Check sheet for the modelled part. Datum: model origin and axes. Units: mm. Face numbers are marked on the shaded views. A direction names the side the tool comes from. Round coordinates to 2 decimals unless told otherwise and drop trailing zeros. Write each loop counter-clockwise with the first axis right and the second up, starting at its lowest first coordinate (ties: lowest second). Pieces come first, ordered by that corner, then holes.
Item 1: Release check for a two-part mould opening along X. For the marked faces 3 and 4 record: pulls with the +X half, pulls with the -X half, needs draft (parallel to the pull), parting line crosses it, or undercut.
Item 2: Section check A-A, the plane z = 4. Record the cut outline in (x, y).
Item 3: Material ranges on line 1 along X through (y, z) = (7, 5.25); line 2 along X through (y, z) = (7, 5.5); line 3 along Y through (x, z) = (-4.5, 3), recorded low to high.
Item 4: Set-up check for the marked faces 1 and 2: record each of +Z, -Z, +X, -X, +Y, -Y from which the full face is reachable in a straight line by a thin tool's end or side.
Item 5: Section check B-B, the plane y = 13. Record the cut outline in (x, z).
Item 6: Depth check by flat-ended pin: pin 1 (1.5 mm diameter, centred on x = 15.5, z = 5, fed in from +Y); pin 2 (1.5 mm diameter, centred on x = -9.5, y = -23.5, fed in from -Z); pin 3 (1.5 mm diameter, centred on y = 1, z = 2, fed in from -X). Enter the tip coordinate at first touch or a pass-through.
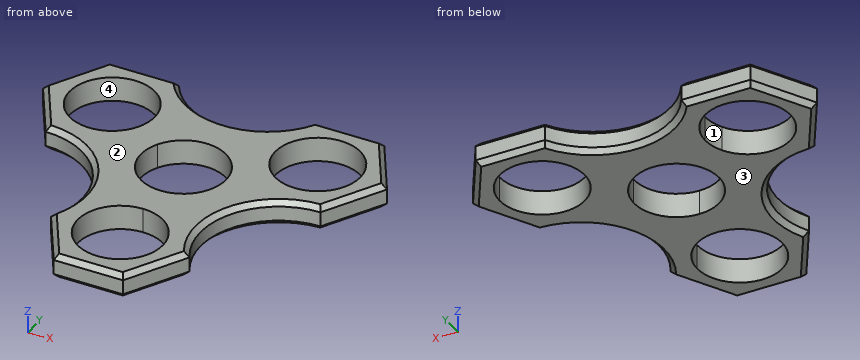
from build123d import *

# Parameters (mm, degrees)
F1_DEPTH = 6.35
F2_SIZE  = 1.27
F3_SIZE  = 1.27


with BuildPart() as f1:
    # F0 (on Top) → F1 (new body)
    with BuildSketch(Plane.XY):
        with BuildLine():
            ThreePointArc((9.535719, 5.50545), (10.635713, 2.849831), (11.0109, 0))
            ThreePointArc((11.0109, 0), (7.785882, -7.785882), (0, -11.0109))
            Line((0, -11.0109), (0, -15.082068))
            Line((0, -15.082068), (8.89, -15.082068))
            Line((8.89, -15.082068), (17.78, -30.48))
            ThreePointArc((17.78, -30.48), (17.78, -10.265288), (35.286454, -0.157932))
            Line((35.286454, -0.157932), (17.506454, -0.157932))
            Line((17.506454, -0.157932), (13.061454, 7.541034))
            Line((13.061454, 7.541034), (9.535719, 5.50545))
        make_face()
        with BuildLine():
            ThreePointArc((-9.535719, 5.50545), (0, 11.0109), (9.535719, 5.50545))
            Line((9.535719, 5.50545), (13.061454, 7.541034))
            Line((13.061454, 7.541034), (8.616454, 15.24))
            Line((8.616454, 15.24), (17.506454, 30.637932))
            ThreePointArc((17.506454, 30.637932), (0, 20.530576), (-17.506454, 30.637932))
            Line((-17.506454, 30.637932), (-8.616454, 15.24))
            Line((-8.616454, 15.24), (-13.061454, 7.541034))
            Line((-13.061454, 7.541034), (-9.535719, 5.50545))
        make_face()
        with BuildLine():
            Line((0, -15.082068), (0, -11.0109))
            ThreePointArc((0, -11.0109), (-9.535719, -5.50545), (-9.535719, 5.50545))
            Line((-9.535719, 5.50545), (-13.061454, 7.541034))
            Line((-13.061454, 7.541034), (-17.506454, -0.157932))
            Line((-17.506454, -0.157932), (-35.286454, -0.157932))
            ThreePointArc((-35.286454, -0.157932), (-17.78, -10.265288), (-17.78, -30.48))
            Line((-17.78, -30.48), (-8.89, -15.082068))
            Line((-8.89, -15.082068), (0, -15.082068))
        make_face()
        with BuildLine():
            ThreePointArc((37.407354, 15.24), (23.546624, 25.875713), (16.860735, 9.73455))
            ThreePointArc((16.860735, 9.73455), (29.246285, 4.604287), (37.407354, 15.24))
        make_face()
        Polygon((8.616454, 15.24), (13.061454, 7.541034), (17.506454, -0.157932), (35.286454, -0.157932), (44.176454, 15.24), (35.286454, 30.637932), (17.506454, 30.637932), align=None)
        with BuildLine():
            ThreePointArc((37.407354, 15.24), (29.246285, 4.604287), (16.860735, 9.73455))
            ThreePointArc((16.860735, 9.73455), (23.546624, 25.875713), (37.407354, 15.24))
        make_face(mode=Mode.SUBTRACT)
        with BuildLine():
            ThreePointArc((11.0109, -30.48), (7.785882, -22.694118), (0, -19.4691))
            ThreePointArc((0, -19.4691), (-7.785882, -38.265882), (11.0109, -30.48))
        make_face()
        Polygon((8.89, -15.082068), (0, -15.082068), (-8.89, -15.082068), (-17.78, -30.48), (-8.89, -45.877932), (8.89, -45.877932), (17.78, -30.48), align=None)
        with BuildLine():
            ThreePointArc((11.0109, -30.48), (-7.785882, -38.265882), (0, -19.4691))
            ThreePointArc((0, -19.4691), (7.785882, -22.694118), (11.0109, -30.48))
        make_face(mode=Mode.SUBTRACT)
        with BuildLine():
            ThreePointArc((-15.385554, 15.24), (-37.032167, 18.089831), (-16.860735, 9.73455))
            ThreePointArc((-16.860735, 9.73455), (-15.760742, 12.390169), (-15.385554, 15.24))
        make_face()
        Polygon((-17.506454, -0.157932), (-13.061454, 7.541034), (-8.616454, 15.24), (-17.506454, 30.637932), (-35.286454, 30.637932), (-44.176454, 15.24), (-35.286454, -0.157932), align=None)
        with BuildLine():
            ThreePointArc((-15.385554, 15.24), (-15.760742, 12.390169), (-16.860735, 9.73455))
            ThreePointArc((-16.860735, 9.73455), (-37.032167, 18.089831), (-15.385554, 15.24))
        make_face(mode=Mode.SUBTRACT)
    extrude(amount=F1_DEPTH)

    # F2
    f2_edges = [f1.edges().sort_by_distance(p)[0] for p in [
        (-26.396454, 30.637932, 6.35),
        (0, 20.530576, 6.35),
        (26.396454, 30.637932, 6.35),
        (39.731454, 22.938966, 6.35),
        (39.731454, 7.541034, 6.35),
        (17.78, -10.265288, 6.35),
        (13.335, -38.178966, 6.35),
        (0, -45.877932, 6.35),
        (-13.335, -38.178966, 6.35),
        (-17.78, -10.265288, 6.35),
        (-39.731454, 7.541034, 6.35),
        (-39.731454, 22.938966, 6.35),
    ]]
    chamfer(f2_edges, length=F2_SIZE)

    # F3
    f3_edges = [f1.edges().sort_by_distance(p)[0] for p in [
        (0, -45.877932, 0),
        (13.335, -38.178966, 0),
        (17.78, -10.265288, 0),
        (39.731454, 7.541034, 0),
        (39.731454, 22.938966, 0),
        (26.396454, 30.637932, 0),
        (0, 20.530576, 0),
        (-26.396454, 30.637932, 0),
        (-39.731454, 22.938966, 0),
        (-39.731454, 7.541034, 0),
        (-17.78, -10.265288, 0),
        (-13.335, -38.178966, 0),
    ]]
    chamfer(f3_edges, length=F3_SIZE)


solid = f1.part
Values found:
1. face 3: needs draft
1. face 4: undercut
2. outline: (-44.18, 15.24) - (-35.29, -0.16) arc R20.21 cw to (-17.78, -30.48) - (-8.89, -45.88) - (8.89, -45.88) - (17.78, -30.48) arc R20.21 cw to (35.29, -0.16) - (44.18, 15.24) - (35.29, 30.64) - (17.51, 30.64) arc R20.21 cw to (-17.51, 30.64) - (-35.29, 30.64) - close; hole (-16.86, 9.73) arc R11.01 ccw to (-15.39, 15.24) arc R11.01 ccw (long way) to start; hole circle Ø22.02 at (0, -30.48); hole (9.54, 5.51) arc R11.01 ccw (long way) to (11.01, 0) arc R11.01 ccw to start; hole circle Ø22.02 at (26.4, 15.24)
3. line 1: x = -39.22 to -33.7, -19.09 to -8.5, 8.5 to 19.09, 33.7 to 39.22
3. line 2: x = -38.93 to -33.7, -19.09 to -8.5, 8.5 to 19.09, 33.7 to 38.93
3. line 3: y = -45.88 to -40.53, -20.43 to -10.05, 10.05 to 21.04
4. face 1: +Z, -Z
4. face 2: +Z, +X, -X, +Y, -Y
5. outline: (-42.88, 1.27) - (-41.42, 0) - (-37.18, 0) - (-37.18, 6.35) - (-41.42, 6.35) - (-42.88, 5.08) - close; (-15.62, 0) - (15.62, 0) - (15.62, 6.35) - (-15.62, 6.35) - close; (37.18, 0) - (41.42, 0) - (42.88, 1.27) - (42.88, 5.08) - (41.42, 6.35) - (37.18, 6.35) - close
6. pin 1: stops at y = 28.72
6. pin 2: stops at z = 0
6. pin 3: stops at x = -36.39
